Here's how the part is built. I have some questions about the finished solid (model axes, mm). A direction names the side the tool comes from. Round coordinates to 2 decimals unless told otherwise and drop trailing zeros. Loops run counter-clockwise (first coordinate to the right, second up) from the corner with the lowest first, then second, coordinate; pieces in that order, holes last. Notation, with made-up numbers: M -11.5,-33.75 L 41.5,-33.75 A20 cw 41.5,-17.75 Z; hole C 86.25,70.5 d1. An arc over 180 degrees is marked long. Put each result on its own line as item: value. Start each with the question number.
```python
from build123d import *

# Parameters (mm, degrees)
ESQCORPS_R   = 8.15
CORPS_DEPTH  = 12
ESQPATTES_R  = 0.5
PATTES_DEPTH = 8
CONG_1_R     = 0.4
ESQDEVANT_R  = 6.55
DEVANT_DEPTH = 0.2


with BuildPart() as part:
    # EsqCorps → Corps (new body)
    with BuildSketch(Plane.XY):
        Circle(ESQCORPS_R)
    extrude(amount=CORPS_DEPTH)

    # EsqPattes → Pattes (add)
    with BuildSketch(Plane(origin=(0, 0, 0), x_dir=(-1, 0, 0), z_dir=(0, 0, -1))):
        with Locations((-5, 0)):
            Circle(ESQPATTES_R)
        with Locations((5, 0)):
            Circle(ESQPATTES_R)
    extrude(amount=PATTES_DEPTH)

    # Congé1
    cong_1_edges = [part.edges().sort_by_distance(p)[0] for p in [
        (-8.15, 0, 0),
        (-8.15, 0, 12),
        (5.5, 0, 0),
        (-4.5, 0, 0),
    ]]
    fillet(cong_1_edges, radius=CONG_1_R)

    # EsqDevant → Devant (cut)
    with BuildSketch(Plane.XY.offset(12)):
        Circle(ESQDEVANT_R)
    extrude(amount=-DEVANT_DEPTH, mode=Mode.SUBTRACT)


solid = part.part
```
1) I'm going to push flat-ended pins straight in: P1, Ø1, axis at x = -5.5, y = -1.5, coming from the +Z side; P2, Ø3, axis at x = -4, z = -2, coming from the +Y side; P3, Ø5, axis at y = 3.5, z = 3, coming from the -X side. Where does each tip first touch, or does it pass through?
2) Suppose I cut it at B-B (x = 0). Write out the boundary of the cut face in (y, z), plus the area to 3 significant figures.
3) Suppose I cut it at A-A (y = 0). Write out the boundary of the cut face in (x, z), plus the area to 3 significant figures.
4) Suppose I cut it at C-C (z = 9). Write out the boundary of the cut face in (x, y), plus the area to 3 significant figures.
5) If we mould it in two halves opening along X, with no side actions, what happens to faces 1 (the face through (5, 0, -8)), 2 (the face through (0, 0, 11.8)), 3 (the face through (5.4, -0.3, -4.1)), 4 (the face through (-6.468, -4.959, 5.922))? For each: pulls with the +X half, pulls with the -X half, needs draft (parallel to the pull), parting line crosses it, or undercut.
6) If I drill on probe 1 along Z at (x, y) = (7.25, -2.75); probe 2 along Z at (x, y) = (0.75, 6.25); probe 3 along X at (y, z) = (-0.25, -1.5), over which ranges is the centre line in solid material (lowest first)? Write a range as from..to.
7) On a 3-axis mill with a long thin cutter (end or side, diameter ignored), from which of +Z, -Z, +X, -X, +Y, -Y can I reach the whole of each face in a straight line? I mean faces 5 (the face through (-4.6, -0.3, -4.1)), 6 (the face through (-5, 0, -8)). Say none if no direction works.
Results are:
1. P1: z = 11.8
1. P2: y = 0.5
1. P3: x = -8.09
2. outline: M -8.15,0.4 A0.4 ccw -7.75,0 L 7.75,0 A0.4 ccw 8.15,0.4 L 8.15,11.6 A0.4 ccw 7.75,12 L 6.55,12 L 6.55,11.8 L -6.55,11.8 L -6.55,12 L -7.75,12 A0.4 ccw -8.15,11.6 Z
2. area: 193 mm²
3. outline: M -8.15,0.4 A0.4 ccw -7.75,0 L -5.9,0 A0.4 cw -5.5,-0.4 L -5.5,-8 L -4.5,-8 L -4.5,-0.4 A0.4 cw -4.1,0 L 4.1,0 A0.4 cw 4.5,-0.4 L 4.5,-8 L 5.5,-8 L 5.5,-0.4 A0.4 cw 5.9,0 L 7.75,0 A0.4 ccw 8.15,0.4 L 8.15,11.6 A0.4 ccw 7.75,12 L 6.55,12 L 6.55,11.8 L -6.55,11.8 L -6.55,12 L -7.75,12 A0.4 ccw -8.15,11.6 Z
3. area: 209 mm²
4. outline: C 0,0 d16.3
4. area: 209 mm²
5. face 1: needs draft
5. face 2: undercut
5. face 3: undercut
5. face 4: parting line crosses it
6. probe 1: 0..12
6. probe 2: 0..11.8
6. probe 3: -5.43..-4.57, 4.57..5.43
7. face 5: -Z
7. face 6: -Z, +X, -X, +Y, -Y
